Read the model definition and answer for the solid it produces. Units are mm, in the model's axes. Face numbers are marked on the shaded views. Give positions to 0.01 mm unless a question says otherwise; leave off trailing zeros. Loops run counter-clockwise (first coordinate to the right, second up) from the corner with the lowest first, then second, coordinate; pieces in that order, holes last. Notation, with made-up numbers: (-30.75, -38.75) -> (-26.75, -38.75) arc R23 cw to (-26.75, 0.25) -> close; hole circle Ø8 at (-2.75, 37.25). An arc over 180 degrees is marked (long way). Write each question's results on one line, items separated by ' | '. Start each with the question number.
Item 1: Find the intervals of material crossed by line 1 (Y direction, x = 0, z = 2.7); line 2 (Y direction, x = 0, z = 1.95), in increasing order.
Item 2: Each of these flat-tipped pins is pushed along its axis until it touches: P1, Ø2, axis at y = -20.5, z = 2, coming from the +X side; P2, Ø2, axis at y = 1.5, z = 2.5, coming from the +X side; P3, Ø2, axis at y = 17.5, z = 1, coming from the +X side. Where does it stop, or does it pass through?
Item 3: Section A-A on y = 0 is taken. Write down the section's boundary in (x, z).
Item 4: Determine the mould class of the marked faces 1 and 2 for opening direction X: +X half, -X half, draft (parallel to the pull), parting line (faces both ways), or undercut.
Item 5: Section D-D on y = -20 is taken. Write down the section's boundary in (x, z), and give its area (3 significant figures).
Item 6: Section C-C on z = 0.65 is taken. Write down the section's boundary in (x, y), and give its area (3 significant figures).
Item 7: Section B-B on x = -3 is taken. Write down the section's boundary in (y, z).
Autodesk Fusion 360 part; units mm, degrees
sketch "Sketch1" plane through (0, 0, 0) normal (0, 0, 1) x (1, 0, 0)
  circle A0 centre (0, 0) radius 31.5
  dimension "d1" = 63
extrude "Extrude1" add sketch "Sketch1" along normal blind 2
sketch "Sketch2" plane through (0, 0, 2) normal (0, 0, 1) x (-1, 0, 0)
  circle A0 centre (0, 0) radius 31.5
  circle A1 centre (0, 0) radius 24.75
  dimension "d4" = 49.5
extrude "Extrude2" add sketch "Sketch2" along normal blind 2 contours A1
sketch "Sketch3" plane through (0, 0, 4) normal (0, 0, 1) x (-1, 0, 0)
  circle A0 centre (0, 0) radius 24.75
  circle A1 centre (0, 0) radius 19
  dimension "d7" = 38
extrude "Extrude3" cut sketch "Sketch3" against normal blind 30 contours A1
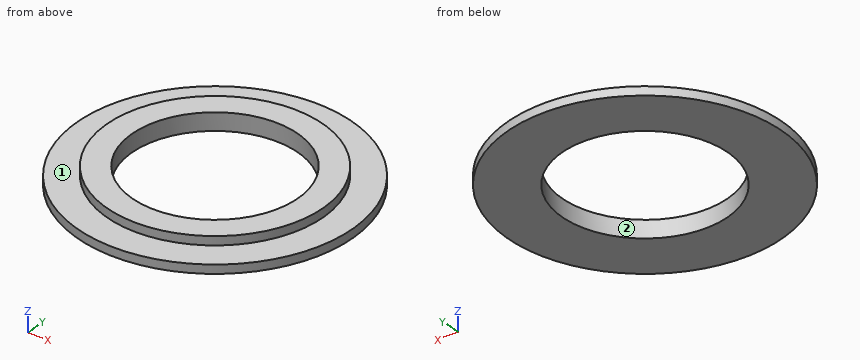
Findings:
1) line 1: -24.75 to -19, 19 to 24.75 | line 2: -31.5 to -19, 19 to 31.5
2) P1: x = 24.74 | P2: x = 31.49 | P3: x = 26.83
3) outline: (-31.5, 0) -> (-19, 0) -> (-19, 4) -> (-24.75, 4) -> (-24.75, 2) -> (-31.5, 2) -> close; (19, 0) -> (31.5, 0) -> (31.5, 2) -> (24.75, 2) -> (24.75, 4) -> (19, 4) -> close
4) face 1: draft | face 2: undercut
5) outline: (-24.34, 0) -> (24.34, 0) -> (24.34, 2) -> (14.58, 2) -> (14.58, 4) -> (-14.58, 4) -> (-14.58, 2) -> (-24.34, 2) -> close | area: 156 mm2
6) outline: circle Ø63 at (0, 0); hole circle Ø38 at (0, 0) | area: 1,980 mm2
7) outline: (-31.36, 0) -> (-18.76, 0) -> (-18.76, 4) -> (-24.57, 4) -> (-24.57, 2) -> (-31.36, 2) -> close; (18.76, 0) -> (31.36, 0) -> (31.36, 2) -> (24.57, 2) -> (24.57, 4) -> (18.76, 4) -> close
